Build history of the part. All positions in model axes, mm. A direction names the side the tool comes from. Give positions to 0.01 mm unless a question says otherwise; leave off trailing zeros. Order: outer loops, then holes, each group sorted by start corner. A loop starts at its lowest first (then second) coordinate and runs counter-clockwise, first axis right, second up. Notation, with made-up numbers: (37.5, -23.75) - (93.5, -23.75) arc R19 cw to (93.5, -12.75) - close; hole circle Ø3 at (-5.5, 88.5). An arc over 180 degrees is marked (long way). Answer in a Markdown table with one row per item.
```python
from build123d import *

# Parameters (mm, degrees)
SKETCH_1_R          = 13.5
EXTRUDE_1_DEPTH     = 10
SKETCH_2_W          = 11.5
SKETCH_2_H          = 60
EXTRUDE_2_DEPTH     = 10
SKETCH_3_R          = 10.25
CUT_EXTRUDE_1_DEPTH = 10
FILLET_1_R          = 10


with BuildPart() as part:
    # 草图1 → 凸台-拉伸1 (new body)
    with BuildSketch(Plane(origin=(0, 0, 0), x_dir=(1, 0, 0), z_dir=(0, 1, 0))):
        with Locations(Location((0, 0, 0), (0, 0, 270))):
            Circle(SKETCH_1_R)
    extrude(amount=EXTRUDE_1_DEPTH)

    # 草图2 → 凸台-拉伸2 (add)
    with BuildSketch(Plane(origin=(0, 10, 0), x_dir=(1, 0, 0), z_dir=(0, 1, 0))):
        Rectangle(SKETCH_2_W, SKETCH_2_H)
    extrude(amount=-EXTRUDE_2_DEPTH)

    # 草图3 → 切除-拉伸1 (cut)
    with BuildSketch(Plane(origin=(0, 10, 0), x_dir=(1, 0, 0), z_dir=(0, 1, 0))):
        with Locations(Location((0, 0, 0), (0, 0, 270))):
            Circle(SKETCH_3_R)
    extrude(amount=-CUT_EXTRUDE_1_DEPTH, mode=Mode.SUBTRACT)

    # 圆角1
    fillet_1_edges = [part.edges().sort_by_distance(p)[0] for p in [
        (-5.75, 5, -12.2142335),
        (-5.75, 5, 12.2142335),
        (5.75, 5, 12.2142335),
        (5.75, 5, -12.2142335),
    ]]
    fillet(fillet_1_edges, radius=FILLET_1_R)


solid = part.part
```
1. Cut at A-A on x = 0. Write the cut outline in (y, z), and give its area (3 significant figures).
Check result:
| item | result |
|---|---|
| outline | (0, -30) - (10, -30) - (10, -10.25) - (0, -10.25) - close; (0, 10.25) - (10, 10.25) - (10, 30) - (0, 30) - close |
| area | 395 mm² |
2. Drop flat-ended pins along their axis: P1, Ø1.5, axis at x = 8, z = -4, coming from the -Y side; P2, Ø4, axis at y = 1.5, z = 13.5, coming from the -X side; P3, Ø5, axis at y = 4, z = -26, coming from the +X side. Give the stop position or say it passes through.
Check result:
| item | result |
|---|---|
| P1 | passes through |
| P2 | stops at x = -7.71 |
| P3 | stops at x = 5.75 |
3. Cut at C-C on z = 0. Write the cut outline in (x, y), and give its area (3 significant figures).
Check result:
| item | result |
|---|---|
| outline | (-13.5, 0) - (-10.25, 0) - (-10.25, 10) - (-13.5, 10) - close; (10.25, 0) - (13.5, 0) - (13.5, 10) - (10.25, 10) - close |
| area | 65.0 mm² |
4. Two-plate mould, pull along Z, no slides. Class faces 1 (the face through (-5.75, 5, 24)), 2 (the face through (0, 5, 30)), 3 (the face through (-10.006, 5.07, -2.222)): +Z half, -Z half, draft (parallel to the pull), parting line (faces both ways), or undercut.
Check result:
| item | result |
|---|---|
| face 1 | draft |
| face 2 | +Z half |
| face 3 | undercut |
5. Cut at D-D on x = -11. Write the cut outline in (y, z).
Check result:
| item | result |
|---|---|
| outline | (0, -7.83) - (10, -7.83) - (10, 7.83) - (0, 7.83) - close |
6. Which spindle directions (+Z, -Z, +X, -X, +Y, -Y) get a long thin tool onto all of the face, cutting with end or side? Do faces 4 (the face through (5.75, 5, -24)), 5 (the face through (5.75, 5, 24)), 6 (the face through (-5.75, 5, -24)), 7 (the face through (-6.59, 4.93, 13.43)). Say none if no direction does.
Check result:
| item | result |
|---|---|
| face 4 | -Z, +X, +Y, -Y |
| face 5 | +Z, +X, +Y, -Y |
| face 6 | -Z, -X, +Y, -Y |
| face 7 | +Z, -X, +Y, -Y |
7. Cut at B-B on y = 9. Write the cut outline in (x, z), and give its area (3 significant figures).
Check result:
| item | result |
|---|---|
| outline | (-9.05, -10.02) arc R10 cw to (-5.75, -17.44) - (-5.75, -30) - (5.75, -30) - (5.75, -17.44) arc R10 cw to (9.05, -10.02) arc R13.5 ccw to (9.05, 10.02) arc R10 cw to (5.75, 17.44) - (5.75, 30) - (-5.75, 30) - (-5.75, 17.44) arc R10 cw to (-9.05, 10.02) arc R13.5 ccw to start; hole circle Ø20.5 at (0, 0) |
| area | 646 mm² |
8. Probe line 1 (Z direction, x = 0.25, y = 6.5); line 2 (X direction, y = 4.25, z = -26); line 3 (Z direction, x = -9.25, y = 2.75). List the from-to ranges inside material, lowest first.
Check result:
| item | result |
|---|---|
| line 1 | z = -30 to -10.25, 10.25 to 30 |
| line 2 | x = -5.75 to 5.75 |
| line 3 | z = -9.83 to -4.42, 4.42 to 9.83 |
